```python
from build123d import *

# Parameters (mm, degrees)
SKETCH1_R                = 17.5
BOSS_EXTRUDE1_DEPTH      = 0.6
CUT_EXTRUDE1_REACH       = 26.756
SKETCH2_R                = 13.5
CUT_EXTRUDE2_REACH       = 26.756
SKETCH3_R                = 1.6
CIRPATTERN1_COUNT        = 6
CIRPATTERN1_ANGLE        = 100
CUT_EXTRUDE3_REACH       = 26.756
SKETCH4_R                = 1.6
CIRPATTERN2_COUNT        = 11
CIRPATTERN2_ANGLE        = 200
F_1_0_1_DIAMETER_HOLE1_D = 1


with BuildPart() as part:
    # Sketch1 → Boss-Extrude1 (new body)
    with BuildSketch(Plane(origin=(0, 0, 0), x_dir=(1, 0, 0), z_dir=(0, 1, 0))):
        with Locations(Location((0, 0, 0), (0, 0, 270))):
            Circle(SKETCH1_R)
    extrude(amount=BOSS_EXTRUDE1_DEPTH)

    # Sketch2 → Cut-Extrude1 (cut, up to next)
    with BuildSketch(Plane(origin=(0, 0.6, 0), x_dir=(1, 0, 0), z_dir=(0, 1, 0)), mode=Mode.PRIVATE) as cut_extrude1_sk1:
        with Locations(Location((0, 0, 0), (0, 0, 270))):
            Circle(SKETCH2_R)
    cut_extrude1_tool1 = extrude(cut_extrude1_sk1.sketch, amount=-CUT_EXTRUDE1_REACH, mode=Mode.PRIVATE) & part.part
    add(cut_extrude1_tool1.solids().sort_by_distance((0, 0.6, 0))[0], mode=Mode.SUBTRACT)

    # Sketch3 → Cut-Extrude2 (cut, up to next)
    with BuildSketch(Plane(origin=(0, 0.6, 0), x_dir=(1, 0, 0), z_dir=(0, 1, 0)), mode=Mode.PRIVATE) as cut_extrude2_sk1:
        with Locations((11.691342951, 6.75)):
            Circle(SKETCH3_R)
    cut_extrude2_tool1 = extrude(cut_extrude2_sk1.sketch, amount=-CUT_EXTRUDE2_REACH, mode=Mode.PRIVATE) & part.part
    cut_extrude2 = cut_extrude2_tool1.solids().sort_by_distance((11.691343, 0.6, -6.75))[0]
    add(cut_extrude2, mode=Mode.SUBTRACT)

    # CirPattern1: Cut-Extrude2 ×6 about axis
    cirpattern1_axis = Axis((0, 0, 0), (0, 1, 0))
    for i in range(1, CIRPATTERN1_COUNT):
        add(cut_extrude2.rotate(cirpattern1_axis, i * CIRPATTERN1_ANGLE / (CIRPATTERN1_COUNT - 1)), mode=Mode.SUBTRACT)

    # Sketch4 → Cut-Extrude3 (cut, up to next)
    with BuildSketch(Plane(origin=(0, 0.6, 0), x_dir=(1, 0, 0), z_dir=(0, 1, 0)), mode=Mode.PRIVATE) as cut_extrude3_sk1:
        with Locations((13.5, 0)):
            Circle(SKETCH4_R)
    cut_extrude3_tool1 = extrude(cut_extrude3_sk1.sketch, amount=-CUT_EXTRUDE3_REACH, mode=Mode.PRIVATE) & part.part
    cut_extrude3 = cut_extrude3_tool1.solids().sort_by_distance((13.5, 0.6, 0))[0]
    add(cut_extrude3, mode=Mode.SUBTRACT)

    # CirPattern2: Cut-Extrude3 ×11 about axis
    cirpattern2_axis = Axis((0, 0, 0), (0, -1, 0))
    for i in range(1, CIRPATTERN2_COUNT):
        add(cut_extrude3.rotate(cirpattern2_axis, i * CIRPATTERN2_ANGLE / (CIRPATTERN2_COUNT - 1)), mode=Mode.SUBTRACT)

    # Ø1.0 (1) Diameter Hole1 (through all)
    with Locations(Plane(origin=(0, 0.6, 0), x_dir=(1, 0, 0), z_dir=(0, 1, 0))):
        with Locations((15.841183551, 4.24463234), (-13.434093526, 9.406653556), (-5.609130351, -15.410958981)):
            Hole(F_1_0_1_DIAMETER_HOLE1_D / 2)


solid = part.part
```
Input: part model. Units: mm. Frame: model coordinates. A direction names the side the tool comes from. Coordinates: 2 decimals unless noted, no trailing zeros. Order: outer loops, then holes, each group sorted by start corner. A loop starts at its lowest first (then second) coordinate and runs counter-clockwise, first axis right, second up. Notation, with made-up numbers: (65, 4.25) - (119, 4.25) arc R11 cw to (119, 10.25) - close; hole circle Ø5 at (21.5, 76). An arc over 180 degrees is marked (long way). Return JSON: item names as keys, results as strings.
Q1. Access query for faces 1 (the cylindrical face through (8.67, 0.3, 10.35)), 2 (the flat face through (-10.3, 0.6, -9.2)). Directions: +Z, -Z, +X, -X, +Y, -Y. A direction counts if a zero-diameter tool reaches every point of the face in a straight line with its end or side. Return the directions, or none.
The answers:
{"face 1": "+Y, -Y", "face 2": "+Z, -Z, +X, -X, +Y"}
Q2. Cut plane C-C (y = 0.3). State how many separate pieces and enclosed holes the cut face has, then the cut area to 3 significant figures.
The answers:
{"separate pieces": "1", "enclosed holes": "4", "area": "317 mm2"}
Q3. Cut plane B-B (z = 0). Return loops of the section in (x, y).
The answers:
{"outline": "(-17.5, 0) - (-15.1, 0) - (-15.1, 0.6) - (-17.5, 0.6) - close; (15.1, 0) - (17.5, 0) - (17.5, 0.6) - (15.1, 0.6) - close"}
Q4. Draft query along Z for faces 3 (the flat face through (-10.3, 0, -9.2)), 4 (the cylindrical face through (13.095, 0.304, -7.518)). Return one class per face: +Z half, -Z half, draft (parallel to the pull), parting line (faces both ways), or undercut.
The answers:
{"face 3": "draft", "face 4": "undercut"}
Q5. Ray query, probe 1 along Z at (x, y) = (11.5, 0.3); probe 2 along X at (y, z) = (0.15, 14.5); probe 3 along X at (y, z) = (0.4, 13). Return the intervals inside material, ascending.
The answers:
{"probe 1": "z = -13.19 to -8.34, 7.07 to 7.57, 9.78 to 13.19", "probe 2": "x = -9.8 to -3.4, -1.29 to 1.29, 3.4 to 9.8", "probe 3": "x = -11.72 to -7.67, -5.83 to -3.92, 3.92 to 5.83, 7.67 to 11.72"}
Q6. Cut plane A-A (x = 0). Return loops of the section in (y, z).
The answers:
{"outline": "(0, -17.5) - (0.6, -17.5) - (0.6, -15.1) - (0, -15.1) - close; (0, 13.5) - (0.6, 13.5) - (0.6, 17.5) - (0, 17.5) - close"}
